from build123d import *

# Parameters (mm, degrees)
SKETCH_1_W          = 150
SKETCH_1_H          = 90
EXTRUDE_1_DEPTH     = 3
SKETCH_2_W          = 90
SKETCH_2_H          = 20
EXTRUDE_2_DEPTH     = 3
SKETCH_3_W          = 90
SKETCH_3_H          = 4
EXTRUDE_3_DEPTH     = 23
CUT_EXTRUDE_1_REACH = 116
SKETCH_4_R          = 2.4


with BuildPart() as part:
    # 스케치1 → 보스-돌출1 (new body)
    with BuildSketch(Plane.XY):
        Rectangle(SKETCH_1_W, SKETCH_1_H)
    extrude(amount=EXTRUDE_1_DEPTH)

    # 스케치2 → 보스-돌출2 (add)
    with BuildSketch(Plane.XY):
        with Locations((0, -55)):
            Rectangle(SKETCH_2_W, SKETCH_2_H)
    extrude(amount=EXTRUDE_2_DEPTH)

    # 스케치3 → 보스-돌출3 (add)
    with BuildSketch(Plane.XY):
        with Locations((0, -67)):
            Rectangle(SKETCH_3_W, SKETCH_3_H)
    extrude(amount=EXTRUDE_3_DEPTH)

    # 스케치4 → 컷-돌출1 (cut, up to next)
    with BuildSketch(Plane.XZ.offset(69), mode=Mode.PRIVATE) as cut_extrude_1_sk1:
        with Locations((-22.5, 13)):
            Circle(SKETCH_4_R)
    cut_extrude_1_tool1 = extrude(cut_extrude_1_sk1.sketch, amount=-CUT_EXTRUDE_1_REACH, mode=Mode.PRIVATE) & part.part
    add(cut_extrude_1_tool1.solids().sort_by_distance((-22.5, -69, 13))[0], mode=Mode.SUBTRACT)
    # 스케치4 → 컷-돌출1 (cut, up to next)
    with BuildSketch(Plane.XZ.offset(69), mode=Mode.PRIVATE) as cut_extrude_1_sk2:
        with Locations((22.5, 13)):
            Circle(SKETCH_4_R)
    cut_extrude_1_tool2 = extrude(cut_extrude_1_sk2.sketch, amount=-CUT_EXTRUDE_1_REACH, mode=Mode.PRIVATE) & part.part
    add(cut_extrude_1_tool2.solids().sort_by_distance((22.5, -69, 13))[0], mode=Mode.SUBTRACT)


solid = part.part
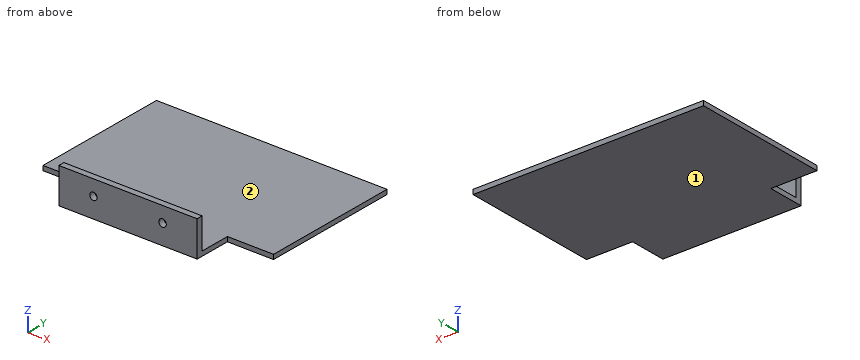
The listing builds one solid part. Answer for the finished solid, in the listing's coordinates (mm). Face numbers are marked on the shaded views. A direction names the side the tool comes from. Coordinates: 2 decimals unless noted, no trailing zeros. Order: outer loops, then holes, each group sorted by start corner. A loop starts at its lowest first (then second) coordinate and runs counter-clockwise, first axis right, second up.
Q1. A cutting plane is placed at A-A, the plane z = 13. Write down the section's boundary in (x, y), and give its area (3 significant figures).
Q2. Which of the six approach directions +Z, -Z, +X, -X, +Y, -Y give full straight-line access (tool end or side, diameter ignored) to the marked faces 1 and 2?
Q3. Consider line 1 (Z direction, x = -22.5, y = -66.85); line 2 (Y direction, x = 14, z = 16.25); line 3 (Z direction, x = -37, y = -51.5). Determine where each line is inside the solid, lowest interval first.
Q4. A cutting plane is placed at B-B, the plane x = -22.5. Write down the section's boundary in (y, z), and give its area (3 significant figures).
Q5. Given P1, Ø0.9, axis at x = 53.5, z = 1, coming from the -Y side; P2, Ø10, axis at x = 19.5, z = 11, coming from the +Y side; P3, Ø4, axis at x = -30.5, y = 27.5, coming from the +Z side, each flat-ended and moving along its own axis, determine where each tip first touches the part or whether it passes through.
Q6. A cutting plane is placed at C-C, the plane y = -40. Write down the section's boundary in (x, z).
Q7. A cutting plane is placed at D-D, the plane x = 33.5. Write down the section's boundary in (y, z).
Answers follow:
1. outline: (-45, -69) - (-24.9, -69) - (-24.9, -65) - (-45, -65) - close; (-20.1, -69) - (20.1, -69) - (20.1, -65) - (-20.1, -65) - close; (24.9, -69) - (45, -69) - (45, -65) - (24.9, -65) - close
1. area: 322 mm2
2. face 1: -Z, +X, -X, +Y, -Y
2. face 2: +Z, +X, -X, +Y
3. line 1: z = 0 to 10.6, 15.4 to 23
3. line 2: y = -69 to -65
3. line 3: z = 0 to 3
4. outline: (-69, 0) - (45, 0) - (45, 3) - (-65, 3) - (-65, 10.6) - (-69, 10.6) - close; (-69, 15.4) - (-65, 15.4) - (-65, 23) - (-69, 23) - close
4. area: 403 mm2
5. P1: stops at y = -45
5. P2: stops at y = -65
5. P3: stops at z = 3
6. outline: (-75, 0) - (75, 0) - (75, 3) - (-75, 3) - close
7. outline: (-69, 0) - (45, 0) - (45, 3) - (-65, 3) - (-65, 23) - (-69, 23) - close
